```python
from build123d import *

# Parameters (mm, degrees)
F0_R     = 25
F0_R_2   = 2.5
F0_R_3   = 5
F1_DEPTH = 5


# Not quite as in the source:
# - a fillet or chamfer that OpenCascade refuses, or shapes differently, is made with other operations: its cross-section is extruded or revolved along the edge and cut away or added


with BuildPart() as f1:
    # F0 (on Front) → F1 (new body)
    with BuildSketch(Plane.XZ):
        Circle(F0_R)
        with Locations((-9.375, -16.237976321)):
            Circle(F0_R_2, mode=Mode.SUBTRACT)
        with Locations((-10.8253175473, -6.25)):
            Circle(F0_R_3, mode=Mode.SUBTRACT)
        with Locations((9.375, -16.237976321)):
            Circle(F0_R_2, mode=Mode.SUBTRACT)
        with Locations((0, -12.5)):
            Circle(F0_R_3, mode=Mode.SUBTRACT)
        with Locations((10.8253175473, -6.25)):
            Circle(F0_R_3, mode=Mode.SUBTRACT)
        with Locations((-18.75, 0)):
            Circle(F0_R_2, mode=Mode.SUBTRACT)
        with Locations((-10.8253175473, 6.25)):
            Circle(F0_R_3, mode=Mode.SUBTRACT)
        with Locations((-9.375, 16.237976321)):
            Circle(F0_R_2, mode=Mode.SUBTRACT)
        with Locations((10.8253175473, 6.25)):
            Circle(F0_R_3, mode=Mode.SUBTRACT)
        with Locations((18.75, 0)):
            Circle(F0_R_2, mode=Mode.SUBTRACT)
        with Locations((0, 12.5)):
            Circle(F0_R_3, mode=Mode.SUBTRACT)
        with Locations((9.375, 16.237976321)):
            Circle(F0_R_2, mode=Mode.SUBTRACT)
    extrude(amount=F1_DEPTH)

    # F3 (on Right) → F5 (revolve, cut)
    with BuildSketch(Plane.YZ):
        with BuildLine():
            Line((-3.5, 25), (-3.5, 24.5))
            ThreePointArc((-3.5, 24.5), (-3.4659258263, 24.7588190451), (-3.3660254038, 25))
            Line((-3.3660254038, 25), (-3.5, 25))
        make_face()
        with BuildLine():
            ThreePointArc((-3.3660254038, 25), (-3.4659258263, 24.7588190451), (-3.5, 24.5))
            ThreePointArc((-3.5, 24.5), (-2.5, 23.5), (-1.5, 24.5))
            ThreePointArc((-1.5, 24.5), (-1.5340741737, 24.7588190451), (-1.6339745962, 25))
            Line((-1.6339745962, 25), (-3.3660254038, 25))
        make_face()
        with BuildLine():
            ThreePointArc((-1.6339745962, 25), (-2.5, 25.5), (-3.3660254038, 25))
            Line((-3.3660254038, 25), (-1.6339745962, 25))
        make_face()
        with BuildLine():
            ThreePointArc((-1.6339745962, 25), (-1.5340741737, 24.7588190451), (-1.5, 24.5))
            Line((-1.5, 24.5), (-1.5, 25))
            Line((-1.5, 25), (-1.6339745962, 25))
        make_face()
    revolve(axis=Axis((0, -2.5, 0), (0, -1, 0)), mode=Mode.SUBTRACT)

    # F6: fillet of radius 5 on 1 edges, made by hand

    # F6_s1 → F6_t2 (revolve, cut)
    with BuildSketch(Plane.XY):
        with BuildLine():
            ThreePointArc((25, -3.5), (23.3657774588, -4.6097722286), (21.4292857857, -5))
            Line((21.4292857857, -5), (25, -5))
            Line((25, -5), (25, -3.5))
        make_face()
    revolve(axis=Axis((0, -5, 0), (0, -1, 0)), mode=Mode.SUBTRACT)


solid = f1.part
```
Work out the finished part from the listing and answer in its coordinate system (mm). A direction names the side the tool comes from. Coordinates: 2 decimals unless noted, no trailing zeros. Write each loop counter-clockwise with the first axis right and the second up, starting at its lowest first coordinate (ties: lowest second). Pieces come first, ordered by that corner, then holes.
Q1. Which of the six approach directions +Z, -Z, +X, -X, +Y, -Y give full straight-line access (tool end or side, diameter ignored) to faces 1 (the face through (0, 0, 0)), 2 (the face through (17, -3.5, 18))?
Q2. Each of these flat-tipped pins is pushed along its axis until it touches: pin 1 Ø2 at (x, y) = (-3.5, -1.5) entering from +Z; pin 2 Ø1 at (x, z) = (-16.5, -17.5) entering from -Y; pin 3 Ø3 at (y, z) = (-2.5, 5) entering from +X. Where does it stop, or does it pass through?
Q3. Determine the mould class of faces 3 (the face through (23.09, -0.74, -9.58)), 4 (the face through (-9.917, -2.465, -18.679)), 5 (the face through (17, -1.5, -18)) for opening direction Z: released by +Z, released by -Z, zero draft, split by the parting line, or undercut.
Q4. A cutting plane is placed at B-B, the plane x = 0. Give the vertices of the cut face in (y, z).
Q5. A cutting plane is placed at A-A, the plane z = 0. Give the vertices of the cut face in (x, y).
Q6. A cutting plane is placed at C-C, the plane z = 14.5. State how many separate pieces and enclosed holes the cut face has, then the cut area to 3 significant figures.
Q7. Find the intervals of material crossed by line 1 (Z direction, x = 0, y = -1.2); line 2 (X direction, y = -2.2, z = -16.5); line 3 (Z direction, x = 8.5, y = -0.5), in increasing order.
Findings below:
1. face 1: +Z, -Z, +X, -X, +Y
1. face 2: none
2. pin 1: stops at z = 24.87
2. pin 2: stops at y = -4.53
2. pin 3: stops at x = 24.7
3. face 3: split by the parting line
3. face 4: undercut
3. face 5: zero draft
4. outline: (-5, -21.43) arc R5 ccw to (-3.5, -25) - (-3.5, -24.5) arc R1 cw to (-1.5, -24.5) - (-1.5, -25) - (0, -25) - (0, -17.5) - (-5, -17.5) - close; (-5, -7.5) - (0, -7.5) - (0, 7.5) - (-5, 7.5) - close; (-5, 17.5) - (0, 17.5) - (0, 25) - (-1.5, 25) - (-1.5, 24.5) arc R1 cw to (-3.5, 24.5) - (-3.5, 25) arc R5 ccw to (-5, 21.43) - close
5. outline: (-25, -3.5) arc R5 ccw to (-21.43, -5) - (-21.25, -5) - (-21.25, 0) - (-25, 0) - (-25, -1.5) - (-24.5, -1.5) arc R1 cw to (-24.5, -3.5) - close; (-16.25, -5) - (16.25, -5) - (16.25, 0) - (-16.25, 0) - close; (21.25, -5) - (21.43, -5) arc R5 ccw to (25, -3.5) - (24.5, -3.5) arc R1 cw to (24.5, -1.5) - (25, -1.5) - (25, 0) - (21.25, 0) - close
6. separate pieces: 4
6. enclosed holes: 0
6. area: 111 mm2
7. line 1: z = -25 to -17.5, -7.5 to 7.5, 17.5 to 25
7. line 2: x = -16.8 to -11.86, -6.89 to -3, 3 to 6.89, 11.86 to 16.8
7. line 3: z = -23.51 to -18.58, -13.9 to -10.68, -1.82 to 1.82, 10.68 to 13.9, 18.58 to 23.51
